Build history of the part. All positions in model axes, mm. Round coordinates to 2 decimals unless told otherwise and drop trailing zeros. Order: outer loops, then holes, each group sorted by start corner. A loop starts at its lowest first (then second) coordinate and runs counter-clockwise, first axis right, second up. Notation, with made-up numbers: M -12,71 L 4,71 A21 ccw 4,76 Z; hole C 36.25,3.5 d2. An arc over 180 degrees is marked long. Use CSV: the item, a comma, the result in double quotes.
from build123d import *

# Parameters (mm, degrees)
SKETCH1_R           = 37.5
SKETCH1_R_2         = 2
BOSS_EXTRUDE1_DEPTH = 3
SKETCH2_R           = 1.35
BOSS_EXTRUDE2_DEPTH = 3
SKETCH2_3_R         = 2
SKETCH2_3_R_2       = 1.35
CUT_EXTRUDE1_DEPTH  = 4
SKETCH3_R           = 20
CUT_EXTRUDE2_DEPTH  = 4


with BuildPart() as part:
    # Sketch1 → Boss-Extrude1 (new body)
    with BuildSketch(Plane(origin=(0, 0, 0), x_dir=(1, 0, 0), z_dir=(0, 1, 0))):
        Circle(SKETCH1_R)
        with Locations((0, 32.5)):
            Circle(SKETCH1_R_2, mode=Mode.SUBTRACT)
        with Locations((28.145825623, 16.25)):
            Circle(SKETCH1_R_2, mode=Mode.SUBTRACT)
        with Locations((28.145825623, -16.25)):
            Circle(SKETCH1_R_2, mode=Mode.SUBTRACT)
        with Locations((0, -32.5)):
            Circle(SKETCH1_R_2, mode=Mode.SUBTRACT)
        with Locations((-28.145825623, -16.25)):
            Circle(SKETCH1_R_2, mode=Mode.SUBTRACT)
        with Locations((-28.145825623, 16.25)):
            Circle(SKETCH1_R_2, mode=Mode.SUBTRACT)
    extrude(amount=BOSS_EXTRUDE1_DEPTH)

    # Sketch2 → Boss-Extrude2 (add, through all)
    with BuildSketch(Plane(origin=(0, 3, 0), x_dir=(1, 0, 0), z_dir=(0, 1, 0))):
        with BuildLine():
            ThreePointArc((-15.1, -34.325500725), (-17.650457715, -33.086422328), (-20.1, -31.6581743))
            Line((-20.1, -31.6581743), (-20.1, -48.1))
            Line((-20.1, -48.1), (20.1, -48.1))
            Line((20.1, -48.1), (20.1, -31.6581743))
            ThreePointArc((20.1, -31.6581743), (17.650457715, -33.086422328), (15.1, -34.325500725))
            Line((15.1, -34.325500725), (15.1, -43.1))
            Line((15.1, -43.1), (-15.1, -43.1))
            Line((-15.1, -43.1), (-15.1, -34.325500725))
        make_face()
        with Locations((-11, -45.3)):
            Circle(SKETCH2_R, mode=Mode.SUBTRACT)
        with Locations((-17.3, -40)):
            Circle(SKETCH2_R, mode=Mode.SUBTRACT)
        with Locations((11, -45.3)):
            Circle(SKETCH2_R, mode=Mode.SUBTRACT)
        with Locations((17.3, -40)):
            Circle(SKETCH2_R, mode=Mode.SUBTRACT)
    extrude(amount=-BOSS_EXTRUDE2_DEPTH)

    # Sketch2<3> → Cut-Extrude1 (cut, through all)
    with BuildSketch(Plane(origin=(0, 3, 0), x_dir=(1, 0, 0), z_dir=(0, 1, 0))):
        with BuildLine():
            Line((15.1, 19), (-15.1, 19))
            Line((-15.1, 19), (-15.1, -34.325500725))
            ThreePointArc((-15.1, -34.325500725), (0, -37.5), (15.1, -34.325500725))
            Line((15.1, -34.325500725), (15.1, 19))
        make_face()
        with Locations((0, -32.5)):
            Circle(SKETCH2_3_R, mode=Mode.SUBTRACT)
        with Locations((-17.3, 4)):
            Circle(SKETCH2_3_R_2)
        with Locations((-17.3, -18)):
            Circle(SKETCH2_3_R_2)
        with Locations((17.3, -18)):
            Circle(SKETCH2_3_R_2)
        with Locations((17.3, 4)):
            Circle(SKETCH2_3_R_2)
    extrude(amount=-CUT_EXTRUDE1_DEPTH, mode=Mode.SUBTRACT)

    # Sketch3 → Cut-Extrude2 (cut, through all)
    with BuildSketch(Plane(origin=(0, 3, 0), x_dir=(1, 0, 0), z_dir=(0, 1, 0))):
        Circle(SKETCH3_R)
    extrude(amount=-CUT_EXTRUDE2_DEPTH, mode=Mode.SUBTRACT)


solid = part.part
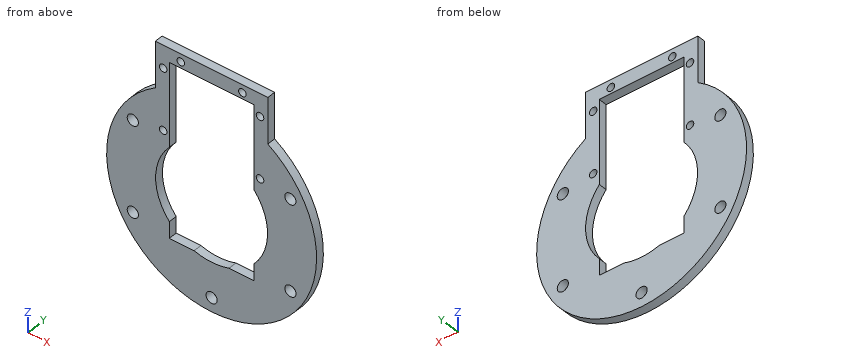
(1) Cut at C-C, the plane x = -11. Give the cut face in (y, z).
Answer block:
outline,"M 0,-35.85 L 3,-35.85 L 3,-19 L 0,-19 Z; M 0,43.1 L 3,43.1 L 3,43.95 L 0,43.95 Z; M 0,46.65 L 3,46.65 L 3,48.1 L 0,48.1 Z"
(2) Drop flat-ended pins along their axis: pin 1 (1.5 mm diameter, centred on x = 1.5, y = 1, fed in from -Z); pin 2 (1.5 mm diameter, centred on y = 1, z = -16, fed in from -X); pin 3 (1.5 mm diameter, centred on y = 1, z = 22.5, fed in from +X). Give the stop position or say it passes through.
Answer block:
pin 1,"stops at z = -37.49"
pin 2,"stops at x = -34.26"
pin 3,"stops at x = 30.55"
(3) Cut at A-A, the plane y = 2.15. Count the separate pieces of the cut face and the enclosed holes in it, and give its area (3 significant figures).
Answer block:
separate pieces,"1"
enclosed holes,"12"
area,"2,760 mm²"
(4) Cut at D-D, the plane x = 14. Give the cut face in (y, z), and give its area (3 significant figures).
Answer block:
outline,"M 0,-34.79 L 3,-34.79 L 3,-19 L 0,-19 Z; M 0,43.1 L 3,43.1 L 3,48.1 L 0,48.1 Z"
area,"62.4 mm²"
(5) Wall check: line 1 (X direction, y = 1.45, z = 40); line 2 (Z direction, x = 11, y = 2.2); line 3 (Z direction, x = 17.3, y = 2.05). Give the ranges that are in metal, low to high. Write a range as from..to.
Answer block:
line 1,"x = -20.1..-18.65, -15.95..-15.1, 15.1..15.95, 18.65..20.1"
line 2,"z = -35.85..-19, 43.1..43.95, 46.65..48.1"
line 3,"z = -33.27..-10.04, 10.04..16.65, 19.35..38.65, 41.35..48.1"
(6) Cut at B-B, the plane z = 36. Give the cut face in (x, y).
Answer block:
outline,"M -20.1,0 L -15.1,0 L -15.1,3 L -20.1,3 Z; M 15.1,0 L 20.1,0 L 20.1,3 L 15.1,3 Z"
